The listing builds one solid part. Answer for the finished solid, in the listing's coordinates (mm). A direction names the side the tool comes from. Coordinates: 2 decimals unless noted, no trailing zeros. Order: outer loops, then holes, each group sorted by start corner. A loop starts at its lowest first (then second) coordinate and runs counter-clockwise, first axis right, second up. Notation, with made-up numbers: (1.25, 36.25) -> (52.25, 36.25) arc R27 ccw to (52.25, 61.25) -> close; hole circle Ø3 at (55.5, 30). An arc over 180 degrees is marked (long way). Return JSON: item names as keys, results as strings.
from build123d import *

# Parameters (mm, degrees)
BOSS_EXTRUDE1_DEPTH = 3
SKETCH2_R           = 0.5
CUT_EXTRUDE1_DEPTH  = 3


with BuildPart() as part:
    # Sketch1 → Boss-Extrude1 (new body)
    with BuildSketch(Plane.XY):
        Polygon((100, -60), (100, -100), (60, -100), (60, -97), (20, -97), (20, -100), (-20, -100), (-20, -97), (-60, -97), (-60, -100), (-100, -100), (-100, -60), (-97, -60), (-97, -20), (-100, -20), (-100, 20), (-97, 20), (-97, 60), (-100, 60), (-100, 100), (-60, 100), (-60, 97), (-20, 97), (-20, 100), (20, 100), (20, 97), (60, 97), (60, 100), (100, 100), (100, 60), (97, 60), (97, 20), (100, 20), (100, -20), (97, -20), (97, -60), align=None)
        with BuildLine():
            ThreePointArc((-57.630385488, -30.062246565), (0, -65), (57.630385488, -30.062246565))
            ThreePointArc((57.630385488, -30.062246565), (52.32882031, -13.198278863), (35.464852608, -18.49984404))
            ThreePointArc((35.464852608, -18.49984404), (0, -40), (-35.464852608, -18.49984404))
            ThreePointArc((-35.464852608, -18.49984404), (-52.32882031, -13.198278863), (-57.630385488, -30.062246565))
        make_face(mode=Mode.SUBTRACT)
        with BuildLine():
            ThreePointArc((35.464852608, 18.49984404), (0, 40), (-35.464852608, 18.49984404))
            ThreePointArc((-35.464852608, 18.49984404), (-52.32882031, 13.198278863), (-57.630385488, 30.062246565))
            ThreePointArc((-57.630385488, 30.062246565), (0, 65), (57.630385488, 30.062246565))
            ThreePointArc((57.630385488, 30.062246565), (52.32882031, 13.198278863), (35.464852608, 18.49984404))
        make_face(mode=Mode.SUBTRACT)
    extrude(amount=BOSS_EXTRUDE1_DEPTH)

    # Sketch2 → Cut-Extrude1 (cut)
    with BuildSketch(Plane.XY.offset(3)):
        with Locations((-13.5, 0)):
            Circle(SKETCH2_R)
        with Locations((-6.75, 11.691342951)):
            Circle(SKETCH2_R)
        with Locations((6.75, 11.691342951)):
            Circle(SKETCH2_R)
        with Locations((13.5, 0)):
            Circle(SKETCH2_R)
        with Locations((6.75, -11.691342951)):
            Circle(SKETCH2_R)
        with Locations((-6.75, -11.691342951)):
            Circle(SKETCH2_R)
    extrude(amount=-CUT_EXTRUDE1_DEPTH, mode=Mode.SUBTRACT)


solid = part.part
1. The part is cut by section D-D on z = 1. Give the number of separate pieces and of enclosed holes in the cut face, and give its area (3 significant figures).
Answer block:
{"separate pieces": "1", "enclosed holes": "8", "area": "32,300 mm2"}
2. Consider line 1 (Y direction, x = -6.75, z = 2.35); line 2 (Y direction, x = 51, z = 1.95); line 3 (X direction, y = 27, z = 0.4). Determine where each line is inside the solid, lowest interval first. Write a range as from..to.
Answer block:
{"line 1": "y = -100..-64.65, -39.43..-12.19, -11.19..11.19, 12.19..39.43, 64.65..100", "line 2": "y = -97..-40.3, -12.6..12.6, 40.3..97", "line 3": "x = -97..-58.75, -29.51..29.51, 58.75..97"}
3. The part is cut by section A-A on y = -45.5. Give the vertices of the cut face in (x, z).
Answer block:
{"outline": "(-97, 0) -> (-46.42, 0) -> (-46.42, 3) -> (-97, 3) -> close; (46.42, 0) -> (97, 0) -> (97, 3) -> (46.42, 3) -> close"}
4. The part is cut by section C-C on y = -24. Give the vertices of the cut face in (x, z), and give its area (3 significant figures).
Answer block:
{"outline": "(-97, 0) -> (-59.04, 0) -> (-59.04, 3) -> (-97, 3) -> close; (-32, 0) -> (32, 0) -> (32, 3) -> (-32, 3) -> close; (59.04, 0) -> (97, 0) -> (97, 3) -> (59.04, 3) -> close", "area": "420 mm2"}
5. For faces 3 (the face through (1, 1, 3)), 4 (the face through (-0.992, -64.992, 1.479)), determine the directions among +Z, -Z, +X, -X, +Y, -Y from which every point of the face is accessible in a straight line to the end or side of a thin tool.
Answer block:
{"face 3": "+Z, +X, -X, +Y, -Y", "face 4": "+Z, -Z"}
6. Determine the mould class of faces 1 (the face through (0.61, -39.995, 1.479)), 2 (the face through (1, 1, 0)) for opening direction Y: pulls with the +Y half, pulls with the -Y half, needs draft (parallel to the pull), parting line crosses it, or undercut.
Answer block:
{"face 1": "undercut", "face 2": "needs draft"}
7. Each of these flat-tipped pins is pushed along its axis until it touches: pin 1 Ø1.5 at (x, z) = (38, 1.5) entering from +Y; pin 2 Ø1.5 at (y, z) = (44, 2.5) entering from -X; pin 3 Ø1.5 at (x, z) = (-46, 1) entering from -Y. Where does it stop, or does it pass through?
Answer block:
{"pin 1": "stops at y = 97", "pin 2": "stops at x = -97", "pin 3": "stops at y = -97"}
8. The part is cut by section B-B on x = 46. Give the vertices of the cut face in (y, z).
Answer block:
{"outline": "(-97, 0) -> (-45.92, 0) -> (-45.92, 3) -> (-97, 3) -> close; (-11.79, 0) -> (11.79, 0) -> (11.79, 3) -> (-11.79, 3) -> close; (45.92, 0) -> (97, 0) -> (97, 3) -> (45.92, 3) -> close"}
